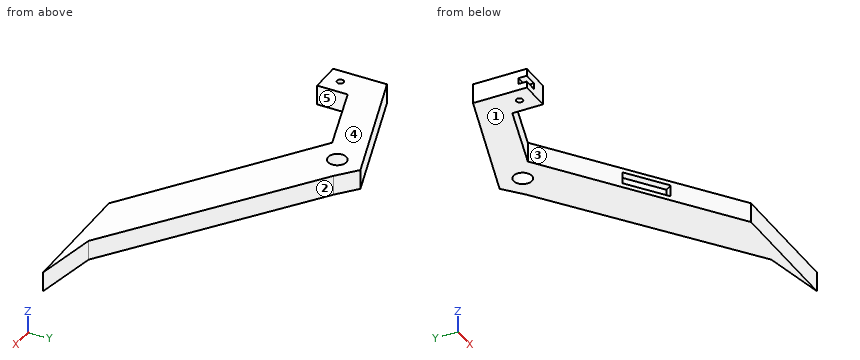
from build123d import *

# Parameters (mm, degrees)
F0_R     = 3.175
F0_R_2   = 8.7650051074
F1_DEPTH = 19.05
F2_W     = 45.4748366028
F2_H     = 11.0821020789
F3_DEPTH = 7.62
F4_W     = 7.8214257956
F4_H     = 5.8546541259
F5_DEPTH = 12.954


with BuildPart() as f1:
    # F0 (on Top) → F1 (new body)
    with BuildSketch(Plane.XY):
        Polygon((177.2020328314, 11.616397533), (-7.5826541561, 148.7761547738), (-25.9976245138, 164.651133018), (-152.9974015162, 123.3761982856), (-152.9974015162, 71.9412896602), (-123.787456631, 71.9412896602), (-123.787456631, 101.1512417973), (-52.0325784639, 124.0111939344), (118.1471256564, 0), (238.161905197, 0), align=None)
        with Locations((-138.3924290736, 86.5462621028)):
            Circle(F0_R, mode=Mode.SUBTRACT)
        with Locations((-31.0776132732, 139.8861721785)):
            Circle(F0_R_2, mode=Mode.SUBTRACT)
    extrude(amount=F1_DEPTH)

    # F2 (on face) → F3 (cut)
    with BuildSketch(Plane(origin=(40.9779427168, 56.2337475009, 0), x_dir=(0.8081842281, -0.5889297526, 0), z_dir=(-0.5889297526, -0.8081842281, 0))):
        with Locations((-3.1541539356, 9.5249998849)):
            Rectangle(F2_W, F2_H)
    extrude(amount=-F3_DEPTH, mode=Mode.SUBTRACT)

    # F4 (on face) → F5 (cut)
    with BuildSketch(Plane(origin=(-152.9974015162, 0, 0), x_dir=(0, -1, 0), z_dir=(-1, 0, 0))):
        with Locations((-75.852002558, 8.9845708571)):
            Rectangle(F4_W, F4_H)
    extrude(amount=-F5_DEPTH, mode=Mode.SUBTRACT)


solid = f1.part
Here's how the part is built. I have some questions about the finished solid (model axes, mm). Face numbers are marked on the shaded views. A direction names the side the tool comes from. Coordinates: 2 decimals unless noted, no trailing zeros. Write each loop counter-clockwise with the first axis right and the second up, starting at its lowest first coordinate (ties: lowest second). Pieces come first, ordered by that corner, then holes. Notation, with made-up numbers: (-34, 47) - (-20, 47) arc R25 ccw to (-20, 77) - close; hole circle Ø2 at (80.25, 46.25). An arc over 180 degrees is marked (long way). Use one line per item in the form item = value.
1) I'm going to push flat-ended pins straight in: P1, Ø9.5, axis at x = -144, z = 9.5, coming from the -Y side; P2, Ø8, axis at y = 51, z = 14.5, coming from the -X side; P3, Ø3, axis at x = -144.5, z = 9, coming from the -Y side. Where does each tip first touch, or does it pass through?
Solved:
P1 = 71.94
P2 = 42.73
P3 = 79.76
2) Suppose I cut it at C-C, the plane y = 41. Write out the boundary of the cut face in (x, z), plus the area to 3 significant figures.
Solved:
outline = (61.88, 0) - (137.62, 0) - (137.62, 19.05) - (61.88, 19.05) - close
area = 1,440 mm2
3) On a 3-axis mill with a long thin cutter (end or side, diameter ignored), from which of +Z, -Z, +X, -X, +Y, -Y can I reach the whole of each face in a straight line? I mean the marked faces 4 and 5. Say none if no direction works.
Solved:
face_4 = +Z, +X, -X, +Y, -Y
face_5 = +Z, -Z, -Y
4) Suppose I cut it at B-B, the plane x = 184. Write out the boundary of the cut face in (y, z), plus the area to 3 significant figures.
Solved:
outline = (0, 0) - (10.32, 0) - (10.32, 19.05) - (0, 19.05) - close
area = 197 mm2
5) Thinking about a two-plate mould opening in X: for the marked faces 1, 2 and 3, which applies, released by +X, released by -X, zero draft, split by the parting line, or undercut?
Solved:
face_1 = zero draft
face_2 = released by +X
face_3 = undercut
6) I need wall thicknesses on line 1 (Y direction, x = -14, z = 15.75); line 2 (Y direction, x = -103, z = 4.5); line 3 (X direction, y = 26, z = 6.75). Which ranges of each line are inside material? Lowest first, please.
Solved:
line_1 = 96.3 to 154.31
line_2 = 107.77 to 139.63
line_3 = 82.47 to 157.82
7) Suppose I cut it at A-A, the plane y = 95.5. Write out the boundary of the cut face in (x, z), plus the area to 3 significant figures.
Solved:
outline = (-153, 0) - (-123.79, 0) - (-123.79, 19.05) - (-153, 19.05) - close; (-12.91, 0) - (64.19, 0) - (64.19, 19.05) - (-12.91, 19.05) - close
area = 2,030 mm2
